Can you work these out from the drawing? Everything is in mm from the part's minimum corner. Coordinates: 2 decimals unless noted, no trailing zeros. Loops run counter-clockwise (first coordinate to the right, second up) from the corner with the lowest first, then second, coordinate; pieces in that order, holes last. Notation, with made-up numbers: M -31,85.25 L 8,85.25 A20 cw 8,90.25 Z; hole C 80,69 d4. An arc over 180 degrees is marked long. Use CSV: the item, a comma, the result in double quotes. Start each with the question number.
Q1. If we section it at C-C (y = 32.5): Please give me the cut outline in (x, z) (1 decimal).
Q2. If we section it at D-D (y = 5): Please give me the cut outline in (x, z).
Q3. If we mould it in two halves opening along Y, with no side actions, what happens to the marked faces 1, 2, 3 and 4? For each: +Y half, -Y half, draft (parallel to the pull), parting line (faces both ways), or undercut.
Q4. If we section it at A-A (x = 16): Please give me the cut outline in (y, z) (1 decimal).
Q5. Please list where these lines run through material, in increasing order: probe 1 along Z at (x, y) = (16, 37.2); probe 2 along Y at (x, z) = (16.5, 35.5) (1 decimal); probe 3 along Y at (x, z) = (13, 36.5) (1 decimal). Write a range as [from, to].
Q6. If we section it at B-B (z = 28): Please give me the cut outline in (x, y), and give its area (3 significant figures).
Q7. For pin 1 Ø7.5 at (x, z) = (16, 19.05) entering from -Y; pin 2 Ø10 at (x, z) = (5, 14) entering from +Y; pin 3 Ø5 at (x, y) = (5.5, 14.5) entering from -Z, each with a flat end and sliding along its axis, tell me the tip position at first contact or that it passes through.
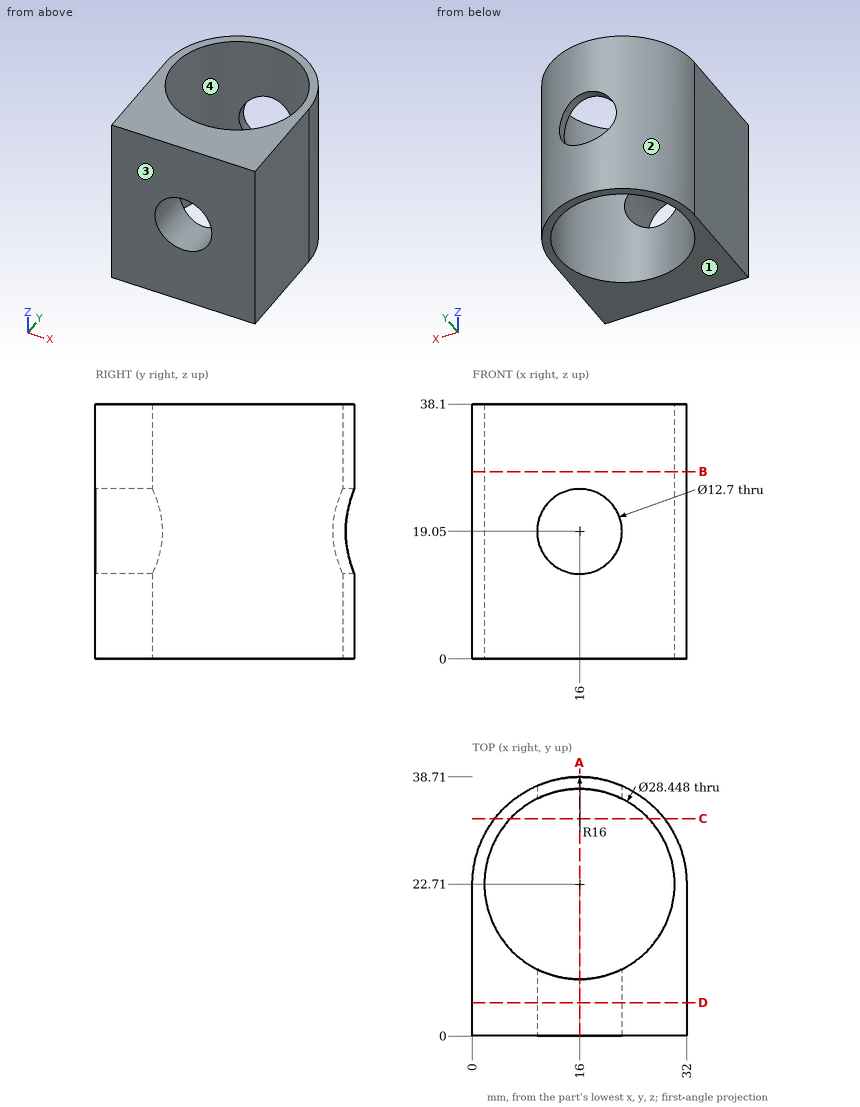
Results below:
1,outline,"M 3.3,0 L 5.7,0 L 5.7,38.1 L 3.3,38.1 Z; M 26.3,0 L 28.7,0 L 28.7,38.1 L 26.3,38.1 Z"
2,outline,"M 0,0 L 32,0 L 32,38.1 L 0,38.1 Z; hole C 16,19.05 d12.7"
3,face 1,"draft"
3,face 2,"+Y half"
3,face 3,"-Y half"
3,face 4,"undercut"
4,outline,"M 0,0 L 8.5,0 L 8.5,12.7 L 0,12.7 Z; M 0,25.4 L 8.5,25.4 L 8.5,38.1 L 0,38.1 Z; M 36.9,0 L 38.7,0 L 38.7,12.7 L 36.9,12.7 Z; M 36.9,25.4 L 38.7,25.4 L 38.7,38.1 L 36.9,38.1 Z"
5,probe 1,"[0, 12.7], [25.4, 38.1]"
5,probe 2,"[0, 8.5], [36.9, 38.7]"
5,probe 3,"[0, 8.8], [36.6, 38.4]"
6,outline,"M 0,0 L 32,0 L 32,22.71 A16 ccw 0,22.71 Z; hole C 16,22.71 d28.45"
6,area,"493 mm^2"
7,pin 1,"through"
7,pin 2,"y = 37.54"
7,pin 3,"z = 0"
